Could you check a few things on this model? Use its own coordinates, in mm. A direction names the side the tool comes from. Give positions to 0.01 mm unless a question says otherwise; leave off trailing zeros. Loops run counter-clockwise (first coordinate to the right, second up) from the corner with the lowest first, then second, coordinate; pieces in that order, holes last.
1. Imagine slicing it at D-D (x = 31). List the corners of the cut face in (y, z) for me, plus the area to 3 significant figures.
2. For P1, Ø6, axis at y = 21, z = 88.5, coming from the +X side; P2, Ø1, axis at y = 24.5, z = 27.5, coming from the -X side; P3, Ø6, axis at y = 21.5, z = 75, coming from the -X side, each with a flat end and sliding along its axis, tell me the tip position at first contact or that it passes through.
3. Imagine slicing it at B-B (z = 24). List the corners of the cut face in (x, y) for me, plus the area to 3 significant figures.
4. Imagine slicing it at A-A (y = 0). List the corners of the cut face in (x, z) for me, plus the area to 3 significant figures.
5. I need wall thicknesses on line 1 along Y through (x, z) = (-1, 16.5); line 2 along X through (y, z) = (21.5, 115.5); line 3 along Y through (x, z) = (20, 126.5). Which ranges of each line are inside material? Lowest first, please.
6. Thinking about a two-plate mould opening in Y: for faces 1 (the cylindrical face through (-30.235, -23.183, 75.133)), 2 (the cylindrical face through (-18.94, 19.18, 131.52)), 3 (the conical face through (3.143, 17.162, 110.764)), which applies, +Y half, -Y half, draft (parallel to the pull), parting line (faces both ways), or undercut?
7. For faces 4 (the cylindrical face through (20.29, -21, 133.08)), 5 (the flat face through (-12.7, 0, 77)), which set-ups out of +Z, -Z, +X, -X, +Y, -Y let a thin tool reach every point of the face, with its end or its side?
8. Imagine slicing it at C-C (z = 142.5). List the corners of the cut face in (x, y) for me (3 decimals).
```python
from build123d import *

# Parameters (mm, degrees)
F0_R           = 38.1
F1_DEPTH       = 152.4
F2_W           = 25.4
F2_H           = 25.4
F3_DEPTH       = 152.4
F5_D           = 6.35
F5_DEPTH       = 38.1
F5_CSINK_D     = 12.7
F5_CSINK_ANGLE = 90
F5_TIP         = 1.9077324654
F7_D           = 10.16
F7_DEPTH       = 38.1
F7_START       = 1.0133538
F7_TIP         = 3.0523719447


with BuildPart() as f1:
    # F0 (on Top) → F1 (new body)
    with BuildSketch(Plane.XY):
        Circle(F0_R)
    extrude(amount=F1_DEPTH)

    # F2 (on face) → F3 (cut, through all)
    with BuildSketch(Plane.XY.offset(152.4)):
        Rectangle(F2_W, F2_H)
    extrude(amount=-F3_DEPTH, mode=Mode.SUBTRACT)

    # F5
    with Locations(Plane.XY.offset(152.4)):
        with Locations((-21.2847962976, -14.3404845148), (-22.1120081842, 19.0418586135), (0, 27.9946457595)):
            CounterSinkHole(F5_D / 2, F5_CSINK_D / 2, depth=F5_DEPTH, counter_sink_angle=F5_CSINK_ANGLE)
            with Locations((0, 0, -(F5_DEPTH + F5_TIP / 2))):  # 118° drill point
                Cone(0, F5_D / 2, F5_TIP, mode=Mode.SUBTRACT)

    # F7
    # its depths count from where the whole tool has entered the part; down to there all is cleared
    with Locations(Plane.XY.offset(152.4)):
        with Locations((2.7354073245, -24.5092585683, 0), (23.9621736109, -24.5092585683, 0), (23.9621736109, 17.9442781955, 0), (2.7354073245, 17.9442781955, -F7_START)):
            Hole(F7_D / 2, depth=F7_DEPTH)
            with Locations((0, 0, -(F7_DEPTH + F7_TIP / 2))):  # 118° drill point
                Cone(0, F7_D / 2, F7_TIP, mode=Mode.SUBTRACT)


solid = f1.part
```
Derived:
1. outline: (-22.15, 0) - (22.15, 0) - (22.15, 152.4) - (-22.15, 152.4) - close
1. area: 6,750 mm2
2. P1: stops at x = 33.58
2. P2: stops at x = -29.59
2. P3: stops at x = -33.31
3. outline: circle Ø76.2 at (0, 0); hole (-12.7, -12.7) - (12.7, -12.7) - (12.7, 12.7) - (-12.7, 12.7) - close
3. area: 3,920 mm2
4. outline: (-38.1, 0) - (-12.7, 0) - (-12.7, 152.4) - (-38.1, 152.4) - close; (12.7, 0) - (38.1, 0) - (38.1, 152.4) - (12.7, 152.4) - close
4. area: 7,740 mm2
5. line 1: y = -38.09 to -12.7, 12.7 to 38.09
5. line 2: x = -31.45 to -24.12, -20.1 to -0.89, 6.36 to 20.33, 27.59 to 31.45
5. line 3: y = -32.43 to -27.69, -21.33 to 14.77, 21.12 to 32.43
6. face 1: parting line
6. face 2: undercut
6. face 3: undercut
7. face 4: +Z
7. face 5: +Z, -Z
8. outline: (24.002, -29.589) arc R5.08 cw (long way) to (29.04, -24.664) arc R38.1 ccw (long way) to start; hole circle Ø6.35 at (-22.112, 19.042); hole circle Ø6.35 at (-21.285, -14.34); hole (-12.7, -12.7) - (12.7, -12.7) - (12.7, 12.7) - (-12.7, 12.7) - close; hole circle Ø6.35 at (0, 27.995); hole circle Ø10.16 at (2.735, -24.509); hole circle Ø10.16 at (2.735, 17.944); hole circle Ø10.16 at (23.962, 17.944)
